from build123d import *

# Parameters (mm, degrees)
F0_R      = 0.9
F1_DEPTH  = 1.8
F2_DEPTH  = 2
F3_W      = 5
F3_H      = 2
F5_DEPTH  = 6.66
F6_R      = 1.8308670993
F7_DEPTH  = 19
F8_R      = 1.25
F9_DEPTH  = 16
F10_DEPTH = 19
F11_R     = 1.8290202659
F11_R_2   = 1.25
F12_DEPTH = 2


with BuildPart() as f1:
    # F0 (on Right) → F1 (new body)
    with BuildSketch(Plane.YZ):
        with BuildLine():
            Line((-19.4736195393, 25.9610565752), (-22.4736195393, 25.9610565752))
            ThreePointArc((-22.4736195393, 25.9610565752), (-23.1807263205, 25.6681633564), (-23.4736195393, 24.9610565752))
            Line((-23.4736195393, 24.9610565752), (-23.4736195393, 15.9610565752))
            Line((-23.4736195393, 15.9610565752), (-18.4736195393, 15.9610565752))
            Line((-18.4736195393, 15.9610565752), (-18.4736195393, 24.9610565752))
            ThreePointArc((-18.4736195393, 24.9610565752), (-18.7665127581, 25.6681633564), (-19.4736195393, 25.9610565752))
        make_face()
        with Locations((-20.9736195393, 24.2594238371)):
            Circle(F0_R, mode=Mode.SUBTRACT)
    extrude(amount=F1_DEPTH)

    # F2 (add): a face of the model
    f2_faces = [f1.faces().sort_by_distance(p)[0] for p in [
        (0.9, -20.9736195393, 15.9610565752),
    ]]
    extrude(f2_faces, amount=F2_DEPTH)


with BuildPart() as f4_1:
    # F4: copy of F1
    add(f1.part.moved(Location((-8.46, 0, 0))))


with BuildPart() as f1_1:
    add(f1.part)

    add(f4_1.part)  # F5 merges F4_1
    # F3 (on face) → F5 (join)
    with BuildSketch(Plane(origin=(0, 0, 0), x_dir=(0, -1, 0), z_dir=(-1, 0, 0))):
        with Locations((20.9736195393, 14.9610565752)):
            Rectangle(F3_W, F3_H)
    extrude(amount=F5_DEPTH)

    # F6 (on face) → F7 (join)
    with BuildSketch(Plane(origin=(0, 0, 13.9610565752), x_dir=(1, 0, 0), z_dir=(0, 0, -1))):
        with Locations((-3.33, 20.9736195393)):
            Circle(F6_R)
    extrude(amount=F7_DEPTH)

    # F8 (on face) → F9 (cut)
    with BuildSketch(Plane.XY.offset(15.9610565752)):
        with Locations((-3.33, -20.9736195393)):
            Circle(F8_R)
    extrude(amount=-F9_DEPTH, mode=Mode.SUBTRACT)

    # F10 (add): a face of the model
    f10_faces = [f1_1.faces().sort_by_distance(p)[0] for p in [
        (-3.33, -23.3594847067, 13.9610565752),
    ]]
    extrude(f10_faces, amount=F10_DEPTH)

    # F11 (on face) → F12 (join)
    with BuildSketch(Plane.XY.offset(15.9610565752)):
        with Locations((-3.33, -20.9736195393)):
            Circle(F11_R)
        with Locations((-3.33, -20.9736195393)):
            Circle(F11_R_2, mode=Mode.SUBTRACT)
    extrude(amount=F12_DEPTH)


solid = f1_1.part
Geometry check sheet. Reference: the model listing, model coordinates, mm. A direction names the side the tool comes from. Give positions to 0.01 mm unless a question says otherwise; leave off trailing zeros. Loops run counter-clockwise (first coordinate to the right, second up) from the corner with the lowest first, then second, coordinate; pieces in that order, holes last.
(1) Section check C-C on z = 7. Record the cut outline in (x, y).
From the geometry:
outline: (-8.46, -23.47) - (1.8, -23.47) - (1.8, -18.47) - (-8.46, -18.47) - close; hole circle Ø2.5 at (-3.33, -20.97)
(2) Section check A-A on x = -3.33. Record the cut outline in (y, z), then the cut area to 3 significant figures.
From the geometry:
outline: (-23.47, -5.04) - (-18.47, -5.04) - (-18.47, 15.96) - (-19.14, 15.96) - (-19.14, 17.96) - (-19.72, 17.96) - (-19.72, -0.04) - (-22.22, -0.04) - (-22.22, 17.96) - (-22.8, 17.96) - (-22.8, 15.96) - (-23.47, 15.96) - close
area: 67.3 mm2
(3) Section check D-D on x = -6.25. Record the cut outline in (y, z).
From the geometry:
outline: (-23.47, -5.04) - (-18.47, -5.04) - (-18.47, 15.96) - (-23.47, 15.96) - close
(4) Set-up check for faces 4 (the flat face through (-3, -21, -0.039)), 5 (the cylindrical face through (-7.57, -23.17, 25.68)), 6 (the flat face through (-2.1, -21.8, 17.961)): record each of +Z, -Z, +X, -X, +Y, -Y from which the full face is reachable in a straight line by a thin tool's end or side.
From the geometry:
face 4: +Z
face 5: +Z, +X, -X, -Y
face 6: +Z, +Y, -Y
(5) Thickness scan on L1, parallel to Z at x = -7.25, y = -21; L2, parallel to X at y = -21.95, z = 19; L3, parallel to Y at x = -3.33, z = 10. Record the ranges inside material, lowest first.
From the geometry:
L1: z = -5.04 to 23.36, 25.16 to 25.96
L2: x = -8.46 to -6.66, 0 to 1.8
L3: y = -23.47 to -22.22, -19.72 to -18.47
(6) Release check for a two-part mould opening along X. For faces 1 (the flat face through (1.8, -21, 11)), 2 (the flat face through (-6.66, -21, 21)), 3 (the flat face through (-3, -18.474, 7)) record: released by +X, released by -X, zero draft, split by the parting line, or undercut.
From the geometry:
face 1: released by +X
face 2: undercut
face 3: zero draft
(7) Section check B-B on y = -20.6. Record the cut outline in (x, z), then the cut area to 3 significant figures.
From the geometry:
outline: (-8.46, -5.04) - (1.8, -5.04) - (1.8, 23.44) - (0, 23.44) - (0, 15.96) - (-1.54, 15.96) - (-1.54, 17.96) - (-2.14, 17.96) - (-2.14, -0.04) - (-4.52, -0.04) - (-4.52, 17.96) - (-5.12, 17.96) - (-5.12, 15.96) - (-6.66, 15.96) - (-6.66, 23.44) - (-8.46, 23.44) - close; (-8.46, 25.08) - (-6.66, 25.08) - (-6.66, 25.96) - (-8.46, 25.96) - close; (0, 25.08) - (1.8, 25.08) - (1.8, 25.96) - (0, 25.96) - close
area: 210 mm2
(8) Depth check by flat-ended pin: pin 1 Ø1.1 at (y, z) = (-20.97, 24.26) entering from +X; pin 2 Ø2.5 at (x, y) = (-2, -22) entering from +Z; pin 3 Ø2 at (y, z) = (-20.97, 24.26) entering from -X. Enter the tip coordinate at first touch or a pass-through.
From the geometry:
pin 1: passes through
pin 2: stops at z = 17.96
pin 3: stops at x = -8.46
